from build123d import *

# Parameters (mm, degrees)
SKETCH1_W                       = 50.8
SKETCH1_H                       = 12.7
BOSS_EXTRUDE1_DEPTH             = 12.7
SKETCH4_R                       = 3.048
CUT_EXTRUDE1_DEPTH              = 50.8
SKETCH6_R                       = 3.175
CUT_EXTRUDE2_DEPTH              = 50.8
TAP_DRILL_FOR_10_24_TAP1_REACH  = 31.099
TAP_DRILL_FOR_10_24_TAP1_BORE_R = 1.89865
FILLET1_R                       = 3.175


with BuildPart() as part:
    # Sketch1 → Boss-Extrude1 (new body)
    with BuildSketch(Plane.XY):
        Rectangle(SKETCH1_W, SKETCH1_H)
    extrude(amount=BOSS_EXTRUDE1_DEPTH)

    # Sketch4 → Cut-Extrude1 (cut)
    with BuildSketch(Plane.XY.offset(12.7)):
        Circle(SKETCH4_R)
    extrude(amount=-CUT_EXTRUDE1_DEPTH, mode=Mode.SUBTRACT)

    # Sketch6 → Cut-Extrude2 (cut)
    with BuildSketch(Plane.XY.offset(12.7)):
        with Locations((19.05, 0)):
            Circle(SKETCH6_R)
    extrude(amount=-CUT_EXTRUDE2_DEPTH, mode=Mode.SUBTRACT)

    # Tap Drill for #10-24 Tap1 bore (on position points) → Tap Drill for #10-24 Tap1 (cut, up to next)
    with BuildSketch(Plane(origin=(0, 6.35, 6.35), x_dir=(1, 0, 0), z_dir=(0, 1, 0)), mode=Mode.PRIVATE) as tap_drill_for_10_24_tap1_sk1:
        Circle(TAP_DRILL_FOR_10_24_TAP1_BORE_R)
    tap_drill_for_10_24_tap1_tool1 = extrude(tap_drill_for_10_24_tap1_sk1.sketch, amount=-TAP_DRILL_FOR_10_24_TAP1_REACH, mode=Mode.PRIVATE) & part.part
    add(tap_drill_for_10_24_tap1_tool1.solids().sort_by_distance((0, 6.35, 6.35))[0], mode=Mode.SUBTRACT)

    # Fillet1
    fillet1_edges = [part.edges().sort_by_distance(p)[0] for p in [
        (-25.4, 6.35, 6.35),
        (25.4, 6.35, 6.35),
        (25.4, -6.35, 6.35),
        (-25.4, -6.35, 6.35),
    ]]
    fillet(fillet1_edges, radius=FILLET1_R)


solid = part.part
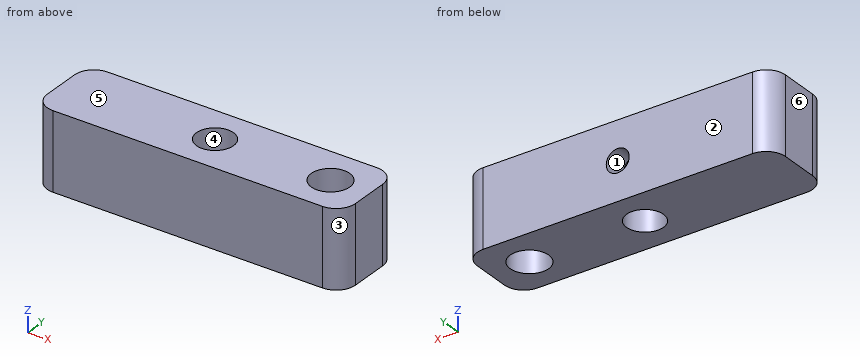
The model under review builds one solid part; all positions refer to its coordinate system, in mm. Face numbers are marked on the shaded views. A direction names the side the tool comes from. Round coordinates to 2 decimals unless told otherwise and drop trailing zeros. Loops run counter-clockwise (first coordinate to the right, second up) from the corner with the lowest first, then second, coordinate; pieces in that order, holes last. Notation, with made-up numbers: (-2.5, -32) -> (21.5, -32) arc R27 ccw to (21.5, -6) -> close; hole circle Ø2 at (35, -12). An arc over 180 degrees is marked (long way). Return JSON: item names as keys, results as strings.
(1) For pin 1 (5 mm diameter, centred on x = 10, y = 4, fed in from -Z); pin 2 (5 mm diameter, centred on x = 19.05, y = 0, fed in from -Z), all flat-tipped, find the tip position at first contact; note any pin that passes through.
Solved:
{"pin 1": "z = 0", "pin 2": "through"}
(2) Add section D-D on x = 0. Write out the cut boundary in (y, z), plus the area to 3 significant figures.
Solved:
{"outline": "(-6.35, 0) -> (-3.05, 0) -> (-3.05, 12.7) -> (-6.35, 12.7) -> close; (3.05, 0) -> (6.35, 0) -> (6.35, 4.45) -> (3.05, 4.45) -> close; (3.05, 8.25) -> (6.35, 8.25) -> (6.35, 12.7) -> (3.05, 12.7) -> close", "area": "71.3 mm2"}
(3) For line 1 (X direction, y = 3.3, z = 6.35); line 2 (X direction, y = -2.75, z = 5.5); line 3 (X direction, y = 1.25, z = 7.75), list the stretches that pass through material, from the lowest coordinate up.
Solved:
{"line 1": "-25.4 to -1.9, 1.9 to 25.4", "line 2": "-25.4 to -1.31, 1.31 to 17.46, 20.64 to 25.4", "line 3": "-25.4 to -2.78, 2.78 to 16.13, 21.97 to 25.4"}
(4) For the marked faces 1 and 2, list the 3-axis set-ups (+Z, -Z, +X, -X, +Y, -Y) from which the entire face can be reached by the end or side of a thin tool; tool diameter is ignored.
Solved:
{"face 1": "+Y", "face 2": "+Z, -Z, +X, -X, +Y"}
(5) The part is to be moulded in two halves that separate along X. For the marked faces 3, 4, 5 and 6, say which applies: released by +X, released by -X, zero draft, split by the parting line, or undercut.
Solved:
{"face 3": "released by +X", "face 4": "undercut", "face 5": "zero draft", "face 6": "released by -X"}
(6) Add section B-B on z = 1.75. Write out the cut boundary in (x, y) (3 decimals).
Solved:
{"outline": "(-25.4, -3.175) arc R3.175 ccw to (-22.225, -6.35) -> (22.225, -6.35) arc R3.175 ccw to (25.4, -3.175) -> (25.4, 3.175) arc R3.175 ccw to (22.225, 6.35) -> (-22.225, 6.35) arc R3.175 ccw to (-25.4, 3.175) -> close; hole circle Ø6.096 at (0, 0); hole circle Ø6.35 at (19.05, 0)"}
(7) Add section A-A on x = 19.05. Write out the cut boundary in (y, z) (3 decimals).
Solved:
{"outline": "(-6.35, 0) -> (-3.175, 0) -> (-3.175, 12.7) -> (-6.35, 12.7) -> close; (3.175, 0) -> (6.35, 0) -> (6.35, 12.7) -> (3.175, 12.7) -> close"}
(8) Add section C-C on y = 0. Write out the cut boundary in (x, z) (3 decimals), plus the area to 3 significant figures.
Solved:
{"outline": "(-25.4, 0) -> (-3.048, 0) -> (-3.048, 12.7) -> (-25.4, 12.7) -> close; (3.048, 0) -> (15.875, 0) -> (15.875, 12.7) -> (3.048, 12.7) -> close; (22.225, 0) -> (25.4, 0) -> (25.4, 12.7) -> (22.225, 12.7) -> close", "area": "487 mm2"}
